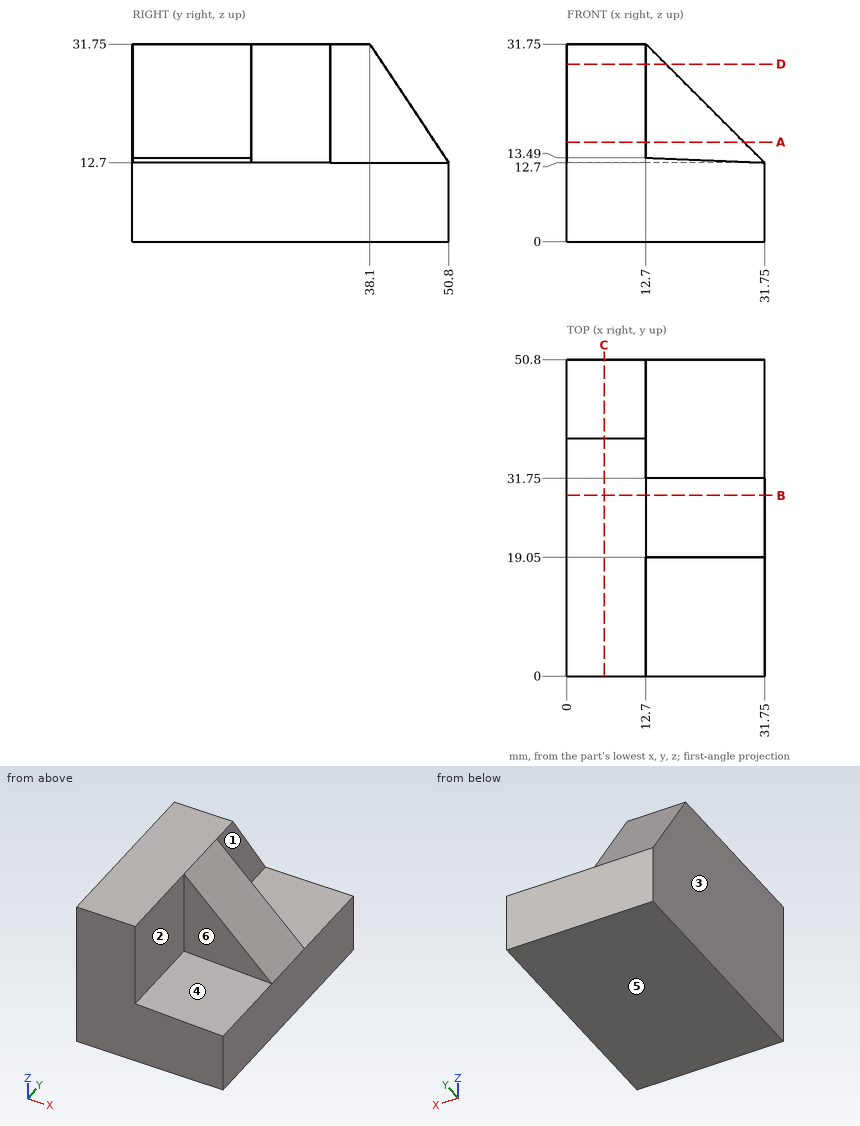
Print and shaded views of the part. All mm, measured from the part's lowest x, y and z. A direction names the side the tool comes from. Coordinates: 2 decimals unless noted, no trailing zeros. Order: outer loops, then holes, each group sorted by start corner. A loop starts at its lowest first (then second) coordinate and runs counter-clockwise, first axis right, second up. Notation, with made-up numbers: (18, 6.5) -> (46, 6.5) arc R28 cw to (46, 35.5) -> close; hole circle Ø8 at (83.5, -38). An arc over 180 degrees is marked (long way). Use one line per item in the form item = value. Start each with the question number.
1) Band-saw the part on B-B on y = 29. Give the cut face in (x, z), then the cut area to 3 significant figures.
2) Drop flat-ended pins along their axis: pin 1 (5.5 mm diameter, centred on y = 12, z = 24.5, fed in from +X); pin 2 (8 mm diameter, centred on x = 13.5, y = 45.5, fed in from -Z); pin 3 (5.5 mm diameter, centred on x = 21, y = 38, fed in from +Z); pin 4 (9.5 mm diameter, centred on x = 17.5, z = 21.5, fed in from -Y). Give the stop position or say it passes through.
3) Tool access for the marked faces 1, 2 and 3: list every direction of +Z, -Z, +X, -X, +Y, -Y with a clear straight run to the whole face (end or side of a thin tool).
4) Band-saw the part on D-D on z = 28.5. Give the cut face in (x, y), then the cut area to 3 significant figures.
5) Band-saw the part on C-C on x = 6. Give the cut face in (y, z), then the cut area to 3 significant figures.
6) Drill centre lines: L1, parallel to X at y = 18.5, z = 20; L2, parallel to Y at x = 13.5, z = 22.5; L3, parallel to Z at x = 1.5, y = 48. Where is each one in solid material? Low to high. Write a range as [from, to].
7) Band-saw the part on A-A on z = 16. Give the cut face in (x, y), then the cut area to 3 significant figures.
8) Pull direction Z, two halves, no side cores. Call the marked faces 4, 5 and 6: +Z half, -Z half, draft (parallel to the pull), parting line (faces both ways), or undercut.
Entries:
q1.outline = (0, 0) -> (31.75, 0) -> (31.75, 12.7) -> (12.7, 31.75) -> (0, 31.75) -> close
q1.area = 827 mm2
q2.pin_1 = 12.7
q2.pin_2 = 0
q2.pin_3 = 12.7
q2.pin_4 = 19.05
q3.face_1 = +Z, +X, +Y
q3.face_2 = +Z, +X, -Y
q3.face_3 = +Z, -Z, -X, +Y, -Y
q4.outline = (0, 0) -> (12.7, 0) -> (12.7, 19.05) -> (15.95, 19.05) -> (15.95, 31.75) -> (12.7, 31.75) -> (12.7, 40.27) -> (0, 40.27) -> close
q4.area = 553 mm2
q5.outline = (0, 0) -> (50.8, 0) -> (50.8, 12.7) -> (38.1, 31.75) -> (0, 31.75) -> close
q5.area = 1,490 mm2
q6.L1 = [0, 12.7]
q6.L2 = [19.05, 31.75]
q6.L3 = [0, 16.9]
q7.outline = (0, 0) -> (12.7, 0) -> (12.7, 19.05) -> (28.45, 19.05) -> (28.45, 31.75) -> (12.7, 31.75) -> (12.7, 48.6) -> (0, 48.6) -> close
q7.area = 817 mm2
q8.face_4 = +Z half
q8.face_5 = -Z half
q8.face_6 = draft
